```python
from build123d import *

# Parameters (mm, degrees)
F0_W     = 118
F0_H     = 70
F1_DEPTH = 28
F2_W     = 10
F2_H     = 70
F3_DEPTH = 25
F4_W     = 23.56403
F4_H     = 9.46647
F5_DEPTH = 5


with BuildPart() as f1:
    # F0 (on Front) → F1 (new body)
    with BuildSketch(Plane.XZ):
        Rectangle(F0_W, F0_H)
    extrude(amount=F1_DEPTH)

    # F2 (on face) → F3 (cut)
    with BuildSketch(Plane.XZ.offset(28)):
        with Locations((54, 0)):
            Rectangle(F2_W, F2_H)
        with Locations((-54, 0)):
            Rectangle(F2_W, F2_H)
    extrude(amount=-F3_DEPTH, mode=Mode.SUBTRACT)

    # F4 (on face) → F5 (join)
    with BuildSketch(Plane(origin=(0, 0, -35), x_dir=(1, 0, 0), z_dir=(0, 0, -1))):
        with BuildLine():
            Line((13.465698, 19.319981), (11.897889, 19.319981))
            ThreePointArc((11.897889, 19.319981), (7.407761, 17.460109), (5.547889, 12.969981))
            Line((5.547889, 12.969981), (5.547889, 11.602327))
            Line((5.547889, 11.602327), (19.815698, 11.602327))
            Line((19.815698, 11.602327), (19.815698, 12.969981))
            ThreePointArc((19.815698, 12.969981), (17.955826, 17.460109), (13.465698, 19.319981))
        make_face()
        with Locations((-19.718742, 14.927268)):
            Rectangle(F4_W, F4_H)
    extrude(amount=F5_DEPTH)


solid = f1.part
```
Check sheet for the modelled part. Datum: model origin and axes. Units: mm. A direction names the side the tool comes from. Round coordinates to 2 decimals unless told otherwise and drop trailing zeros. Order: outer loops, then holes, each group sorted by start corner. A loop starts at its lowest first (then second) coordinate and runs counter-clockwise, first axis right, second up. Notation, with made-up numbers: (16, 18.25) -> (40, 18.25) arc R32 ccw to (40, 50.25) -> close; hole circle Ø10 at (-32.5, 54.25). An arc over 180 degrees is marked (long way). One line per item, written item: value. Start each with the question number.
Q1. Gauge pin test, flat ends, axial feed: pin 1 Ø1.5 at (x, z) = (-22.5, -36.5) entering from -Y; pin 2 Ø10 at (y, z) = (-17, 22) entering from -X; pin 3 Ø6 at (x, y) = (43, -7) entering from -Z. Record the tip position at first contact, or that the pin passes through.
Q2. Cross-section at C-C (x = 52). Record the boundary of the cut face in (y, z).
Q3. Cross-section at A-A (z = 6.5). Record the boundary of the cut face in (x, y), and give its area (3 significant figures).
Q4. Thickness scan on line 1 (X direction, y = -25.25, z = -17.5); line 2 (Z direction, x = 8, y = -22.25). Record the ranges inside material, lowest first.
Q5. Set-up check for faces 1 (the face through (-7.937, -15, -37)), 2 (the face through (49, -16, 0)), 3 (the face through (-54, -3, 0)), 4 (the face through (18.005, -17.41, -37.465)), 5 (the face through (13, -11.602, -37)): record each of +Z, -Z, +X, -X, +Y, -Y from which the full face is reachable in a straight line by a thin tool's end or side.
Q6. Cross-section at B-B (y = -14.25). Record the boundary of the cut face in (x, z).
Q7. Cross-section at D-D (y = -6.5). Record the boundary of the cut face in (x, z).
Completed:
1. pin 1: stops at y = -19.66
1. pin 2: stops at x = -49
1. pin 3: stops at z = -35
2. outline: (-3, -35) -> (0, -35) -> (0, 35) -> (-3, 35) -> close
3. outline: (-59, -3) -> (-49, -3) -> (-49, -28) -> (49, -28) -> (49, -3) -> (59, -3) -> (59, 0) -> (-59, 0) -> close
3. area: 2,800 mm²
4. line 1: x = -49 to 49
4. line 2: z = -35 to 35
5. face 1: -Z, +Y, -Y
5. face 2: +Z, -Z, +X, -Y
5. face 3: +Z, -Z, -X, -Y
5. face 4: -Z, +X, -Y
5. face 5: -Z, +X, +Y
6. outline: (-49, -35) -> (-31.5, -35) -> (-31.5, -40) -> (-7.94, -40) -> (-7.94, -35) -> (5.68, -35) -> (5.68, -40) -> (19.69, -40) -> (19.69, -35) -> (49, -35) -> (49, 35) -> (-49, 35) -> close
7. outline: (-49, -35) -> (49, -35) -> (49, 35) -> (-49, 35) -> close
